from build123d import *

# Parameters (mm, degrees)
F0_R     = 1.9
F0_W     = 4
F0_H     = 21
F1_DEPTH = 4
F2_W     = 26
F2_H     = 28
F2_W_2   = 22
F2_H_2   = 24
F3_DEPTH = 8
F5_D     = 1
F6_DEPTH = 4


with BuildPart() as f1:
    # F0 (on Top) → F1 (new body)
    with BuildSketch(Plane.XY):
        with BuildLine():
            ThreePointArc((20, 12.5), (18.5355339059, 16.0355339059), (15, 17.5))
            Line((15, 17.5), (-15, 17.5))
            ThreePointArc((-15, 17.5), (-18.5355339059, 16.0355339059), (-20, 12.5))
            Line((-20, 12.5), (-20, -12.5))
            ThreePointArc((-20, -12.5), (-18.5355339059, -16.0355339059), (-15, -17.5))
            Line((-15, -17.5), (15, -17.5))
            ThreePointArc((15, -17.5), (18.5355339059, -16.0355339059), (20, -12.5))
            Line((20, -12.5), (20, 12.5))
        make_face()
        with Locations((-16, -8)):
            Circle(F0_R, mode=Mode.SUBTRACT)
        with Locations((16, -8)):
            Circle(F0_R, mode=Mode.SUBTRACT)
        with Locations((-16, 8)):
            Circle(F0_R, mode=Mode.SUBTRACT)
        with Locations((-8, 1.1)):
            Rectangle(F0_W, F0_H, mode=Mode.SUBTRACT)
        with Locations((16, 8)):
            Circle(F0_R, mode=Mode.SUBTRACT)
    extrude(amount=F1_DEPTH)

    # F2 (on face) → F3 (join)
    with BuildSketch(Plane.XY.offset(4)):
        Rectangle(F2_W, F2_H)
        Rectangle(F2_W_2, F2_H_2, mode=Mode.SUBTRACT)
    extrude(amount=F3_DEPTH)

    # F5 (through all)
    with Locations(Plane.XY.offset(4)):
        with Locations((-3.64, -9.36), (8.36, -9.36), (8.36, 7.64), (-3.64, 7.64)):
            Hole(F5_D / 2)

    # F6 (add): a face of the model
    f6_faces = [f1.faces().sort_by_distance(p)[0] for p in [
        (1.5074813824, -0.2034626738, 4),
    ]]
    extrude(f6_faces, amount=F6_DEPTH)


solid = f1.part
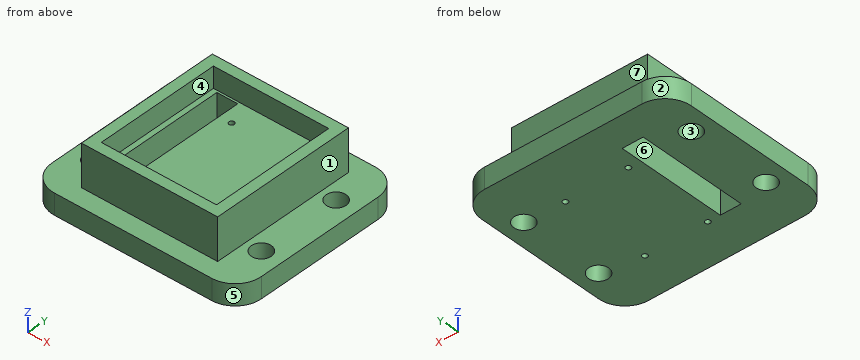
For this review, take the finished solid that the model builds, in its own axes (mm). Face numbers are marked on the shaded views. A direction names the side the tool comes from. Coordinates: 2 decimals unless noted, no trailing zeros. Write each loop counter-clockwise with the first axis right and the second up, starting at its lowest first coordinate (ties: lowest second). Pieces come first, ordered by that corner, then holes. Notation, with made-up numbers: (48.25, 84.5) -> (65.25, 84.5) arc R29 ccw to (65.25, 113.5) -> close; hole circle Ø3 at (80, -5.5). An arc over 180 degrees is marked (long way). Write each question's results on one line, items separated by ' | '. Start each with the question number.
1) The part is to be moulded in two halves that separate along Y. For the marked faces 1, 2 and 3, say which applies: +Y half, -Y half, draft (parallel to the pull), parting line (faces both ways), or undercut.
2) For the marked faces 4, 5, 6 and 7, list the 3-axis set-ups (+Z, -Z, +X, -X, +Y, -Y) from which the entire face can be reached by the end or side of a thin tool; tool diameter is ignored.
3) Insertion check: pin 1 (2 mm diameter, centred on x = 0, z = 11, fed in from +Y); pin 2 (1.2 mm diameter, centred on y = -3.5, z = 10.5, fed in from +X); pin 3 (2.5 mm diameter, centred on x = 16, y = -8, fed in from -Z); pin 4 (17.5 mm diameter, centred on x = -1.5, y = 1, fed in from +Z). Each pin has a flat end and moves straight along its axis. Give the tip position at first contact, or say it passes through.
4) Consider section B-B (y = -8). Write out the cut boundary in (x, z), plus the area to 3 significant figures.
5) Consider section D-D (y = 5.5). Write out the cut boundary in (x, z).
6) Consider section A-A (z = 8.75). Write out the cut boundary in (x, y).
7) Consider section C-C (x = 8.36). Write out the cut boundary in (y, z).
8) Wall thickness on L1, parallel to Y at x = 8.36, z = 3.25; L2, parallel to Y at x = -7, z = 10.5; L3, parallel to X at y = 3, z = 1.5: over which ranges is each line inside the solid? List them lowest first. Write a range as [from, to].
Geometry says:
1) face 1: draft | face 2: +Y half | face 3: undercut
2) face 4: +Z | face 5: +Z, -Z, +X, -Y | face 6: +Z, -Z | face 7: +Z, +X, -X, +Y
3) pin 1: y = 14 | pin 2: x = 13 | pin 3: through | pin 4: z = 8
4) outline: (-20, 0) -> (-17.9, 0) -> (-17.9, 4) -> (-20, 4) -> close; (-14.1, 0) -> (-10, 0) -> (-10, 8) -> (-11, 8) -> (-11, 12) -> (-13, 12) -> (-13, 4) -> (-14.1, 4) -> close; (-6, 0) -> (14.1, 0) -> (14.1, 4) -> (13, 4) -> (13, 12) -> (11, 12) -> (11, 8) -> (-6, 8) -> close; (17.9, 0) -> (20, 0) -> (20, 4) -> (17.9, 4) -> close | area: 218 mm^2
5) outline: (-20, 0) -> (-10, 0) -> (-10, 8) -> (-11, 8) -> (-11, 12) -> (-13, 12) -> (-13, 4) -> (-20, 4) -> close; (-6, 0) -> (20, 0) -> (20, 4) -> (13, 4) -> (13, 12) -> (11, 12) -> (11, 8) -> (-6, 8) -> close
6) outline: (-13, -14) -> (13, -14) -> (13, 14) -> (-13, 14) -> close; hole (-11, -12) -> (11, -12) -> (11, 12) -> (-11, 12) -> close
7) outline: (-17.5, 0) -> (-9.86, 0) -> (-9.86, 8) -> (-12, 8) -> (-12, 12) -> (-14, 12) -> (-14, 4) -> (-17.5, 4) -> close; (-8.86, 0) -> (7.14, 0) -> (7.14, 8) -> (-8.86, 8) -> close; (8.14, 0) -> (17.5, 0) -> (17.5, 4) -> (14, 4) -> (14, 12) -> (12, 12) -> (12, 8) -> (8.14, 8) -> close
8) L1: [-17.5, -9.86], [-8.86, 7.14], [8.14, 17.5] | L2: [-14, -12], [12, 14] | L3: [-20, -10], [-6, 20]
